Part print with two shaded views. Sizes in mm from the minimum x, y, z corner. A direction names the side the tool comes from. Round coordinates to 2 decimals unless told otherwise and drop trailing zeros. Write each loop counter-clockwise with the first axis right and the second up, starting at its lowest first coordinate (ties: lowest second). Pieces come first, ordered by that corner, then holes. Notation, with made-up numbers: M -39,50.25 L -32,50.25 A20 ccw -32,67.25 Z; hole C 77,32 d11. An arc over 180 degrees is marked long. Use one line per item in the form item = value. Start each with the question number.
Item 1: Mould opens along X. For the marked faces 6, 7 and 8 say: +X half, -X half, draft (parallel to the pull), parting line (faces both ways), or undercut.
Item 2: Cut at A-A, the plane y = 2. Give the cut face in (x, z).
Item 3: Cut at C-C, the plane z = 10. Give the cut face in (x, y), then the cut area to 3 significant figures.
Item 4: Flat gauge pins, fed straight in: pin 1 Ø1 at (y, z) = (3, 5) entering from -X; pin 2 Ø5 at (x, y) = (14, 4) entering from +Z; pin 3 Ø5.5 at (x, z) = (5.5, 6.5) entering from -Y; pin 4 Ø1.8 at (y, z) = (7.5, 5.5) entering from +X. Where does each tip first touch, or does it go through?
Item 5: Which spindle directions (+Z, -Z, +X, -X, +Y, -Y) get a long thin tool onto all of the face, cutting with end or side? Do the marked faces 1, 2, 3, 4 and 5. Say none if no direction does.
Item 6: Probe L1, parallel to Y at x = 2, z = 8; L2, parallel to Y at x = 6.25, z = 8.75; L3, parallel to X at y = 4.25, z = 9.25. List the from-to ranges inside material, lowest first.
Item 7: Cut at B-B, the plane x = 3.9. Give the cut face in (y, z), then the cut area to 3 significant figures.
Item 8: Cut at D-D, the plane z = 5.2. Give the cut face in (x, y).
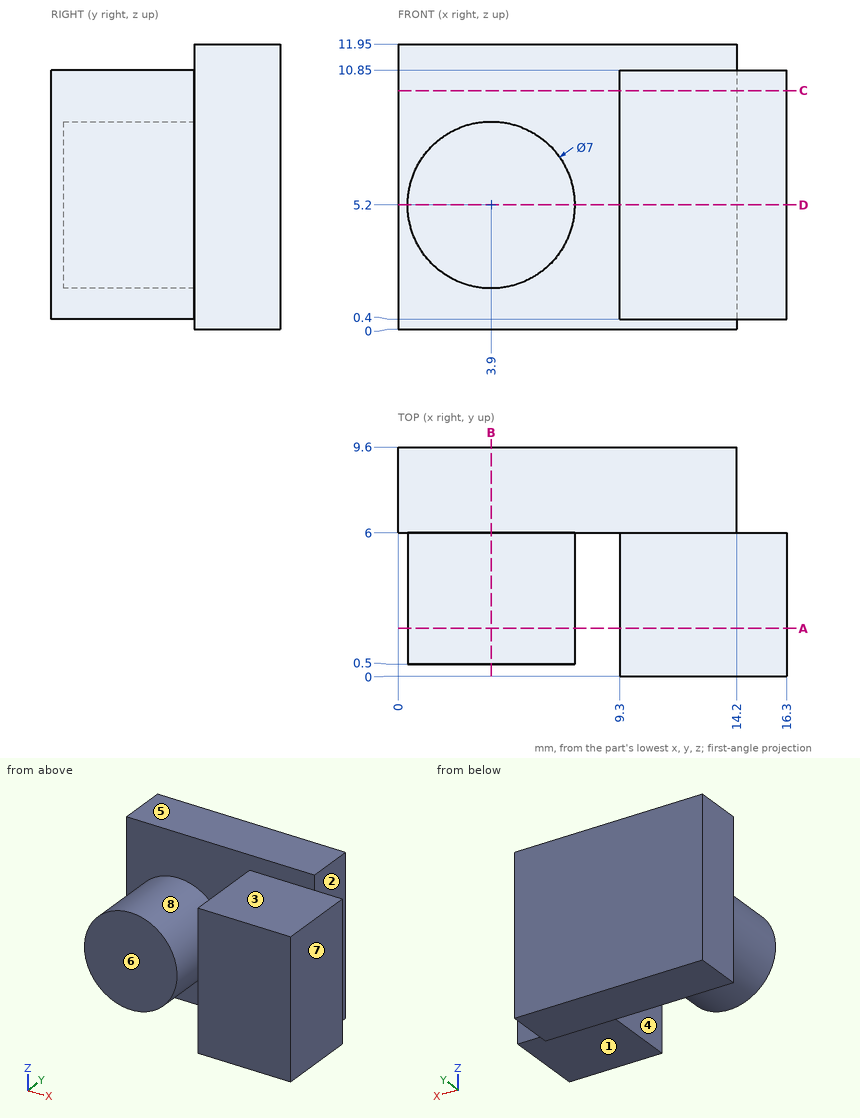
Model answer:
q1.face_6 = draft
q1.face_7 = +X half
q1.face_8 = undercut
q2.outline = C 3.9,5.2 d7; M 9.3,0.4 L 16.3,0.4 L 16.3,10.85 L 9.3,10.85 Z
q3.outline = M 0,6 L 9.3,6 L 9.3,0 L 16.3,0 L 16.3,6 L 14.2,6 L 14.2,9.6 L 0,9.6 Z
q3.area = 93.1 mm²
q4.pin_1 = 0.4
q4.pin_2 = 11.95
q4.pin_3 = 0.5
q4.pin_4 = 14.2
q5.face_1 = -Z, +X, -X, -Y
q5.face_2 = +Z, -Z, +X, +Y
q5.face_3 = +Z, +X, -X, -Y
q5.face_4 = +Z, -Z, -Y
q5.face_5 = +Z, +X, -X, +Y, -Y
q6.L1 = 0.5 to 9.6
q6.L2 = 6 to 9.6
q6.L3 = 9.3 to 16.3
q7.outline = M 0.5,1.7 L 6,1.7 L 6,0 L 9.6,0 L 9.6,11.95 L 6,11.95 L 6,8.7 L 0.5,8.7 Z
q7.area = 81.5 mm²
q8.outline = M 0,6 L 0.4,6 L 0.4,0.5 L 7.4,0.5 L 7.4,6 L 9.3,6 L 9.3,0 L 16.3,0 L 16.3,6 L 14.2,6 L 14.2,9.6 L 0,9.6 Z
